from build123d import *

# Parameters (mm, degrees)
F0_W     = 38.1
F0_H     = 1219.2
F1_DEPTH = 19.05
F2_R     = 12.7
F3_DEPTH = 25
F4_R     = 6.35
F4_R_2   = 12.7
F5_DEPTH = 25


with BuildPart() as f1:
    # F0 (on Front) → F1 (new body)
    with BuildSketch(Plane.XZ):
        with Locations((19.05, 609.6)):
            Rectangle(F0_W, F0_H)
    extrude(amount=F1_DEPTH)

    # F2 (on face) → F3 (cut)
    with BuildSketch(Plane.XZ.offset(19.05)):
        with Locations((19.05, 400)):
            Circle(F2_R)
    extrude(amount=-F3_DEPTH, mode=Mode.SUBTRACT)

    # F4 (on face) → F5 (cut)
    with BuildSketch(Plane.XZ.offset(19.05)):
        with Locations((19.05, 1194.2)):
            Circle(F4_R)
        with Locations((19.05, 25)):
            Circle(F4_R_2)
    extrude(amount=-F5_DEPTH, mode=Mode.SUBTRACT)


solid = f1.part
Design review of the part built by this model. Coordinates are the model's own, in mm. Round coordinates to 2 decimals unless told otherwise and drop trailing zeros. Write each loop counter-clockwise with the first axis right and the second up, starting at its lowest first coordinate (ties: lowest second). Pieces come first, ordered by that corner, then holes. Notation, with made-up numbers: (2, 3.5) -> (59, 3.5) arc R11 cw to (59, 14.5) -> close; hole circle Ø1 at (35, 25). An arc over 180 degrees is marked (long way). One line per item, written item: value. Start each with the question number.
Q1. Add section A-A (z = 400). Give the boundary of the cut face in (x, y), then the cut area to 3 significant figures.
Q2. Add section C-C (y = -10). Give the boundary of the cut face in (x, z).
Q3. Add section B-B (x = 19.05). Give the boundary of the cut face in (y, z).
Q4. The part is to be moulded in two halves that separate along X. For faces 1 (the face through (38.1, -9, 601)), 2 (the face through (31.164, -9.658, 28.815)), 3 (the face through (19, 0, 618)), say which applies: pulls with the +X half, pulls with the -X half, needs draft (parallel to the pull), parting line crosses it, or undercut.
Q5. To check wall thickness, follow probe 1 along Z at (x, y) = (19.05, -14.25); probe 2 along Z at (x, y) = (29, -13.5); probe 3 along Z at (x, y) = (22, -3.5). State the ranges of each line that lie inside material, in increasing order.
Response:
1. outline: (0, -19.05) -> (6.35, -19.05) -> (6.35, 0) -> (0, 0) -> close; (31.75, -19.05) -> (38.1, -19.05) -> (38.1, 0) -> (31.75, 0) -> close
1. area: 242 mm^2
2. outline: (0, 0) -> (38.1, 0) -> (38.1, 1219.2) -> (0, 1219.2) -> close; hole circle Ø25.4 at (19.05, 25); hole circle Ø25.4 at (19.05, 400); hole circle Ø12.7 at (19.05, 1194.2)
3. outline: (-19.05, 0) -> (0, 0) -> (0, 12.3) -> (-19.05, 12.3) -> close; (-19.05, 37.7) -> (0, 37.7) -> (0, 387.3) -> (-19.05, 387.3) -> close; (-19.05, 412.7) -> (0, 412.7) -> (0, 1187.85) -> (-19.05, 1187.85) -> close; (-19.05, 1200.55) -> (0, 1200.55) -> (0, 1219.2) -> (-19.05, 1219.2) -> close
4. face 1: pulls with the +X half
4. face 2: undercut
4. face 3: needs draft
5. probe 1: z = 0 to 12.3, 37.7 to 387.3, 412.7 to 1187.85, 1200.55 to 1219.2
5. probe 2: z = 0 to 17.11, 32.89 to 392.11, 407.89 to 1219.2
5. probe 3: z = 0 to 12.65, 37.35 to 387.65, 412.35 to 1188.58, 1199.82 to 1219.2
